```python
from build123d import *

# Parameters (mm, degrees)
SK_P01_P2020_R  = 2.1
P01_P2020_DEPTH = 120


with BuildPart() as part:
    # SK_P01_p2020 → P01_p2020 (new body)
    with BuildSketch(Plane(origin=(0, 0, 0), x_dir=(1, 0, 0), z_dir=(0, 1, 0))):
        Polygon((10, -10), (10, -3.1), (4, -3.1), (4, 3.1), (10, 3.1), (10, 10), (3.1, 10), (3.1, 4), (-3.1, 4), (-3.1, 10), (-10, 10), (-10, 3.1), (-4, 3.1), (-4, -3.1), (-10, -3.1), (-10, -10), (-3.1, -10), (-3.1, -4), (3.1, -4), (3.1, -10), align=None)
        with Locations(Location((0, 0, 0), (0, 0, 270))):
            Circle(SK_P01_P2020_R, mode=Mode.SUBTRACT)
    extrude(amount=P01_P2020_DEPTH)


solid = part.part
```
Here's how the part is built. I have some questions about the finished solid (model axes, mm). A direction names the side the tool comes from. Coordinates: 2 decimals unless noted, no trailing zeros. Order: outer loops, then holes, each group sorted by start corner. A loop starts at its lowest first (then second) coordinate and runs counter-clockwise, first axis right, second up. Notation, with made-up numbers: (55.5, 23) -> (90.5, 23) arc R30 cw to (90.5, 57) -> close; hole circle Ø1 at (-3, -37). An arc over 180 degrees is marked (long way). Return JSON: item names as keys, results as strings.
1) If we section it at B-B on z = -6.25: List the corners of the cut face in (x, y) for me.
Conclusion:
{"outline": "(-10, 0) -> (-3.1, 0) -> (-3.1, 120) -> (-10, 120) -> close; (3.1, 0) -> (10, 0) -> (10, 120) -> (3.1, 120) -> close"}
2) If I drill on probe 1 along Z at (x, y) = (-7.75, 58); probe 2 along X at (y, z) = (51.5, 0), over which ranges is the centre line in solid material (lowest first)?
Conclusion:
{"probe 1": "z = -10 to -3.1, 3.1 to 10", "probe 2": "x = -4 to -2.1, 2.1 to 4"}
3) If we section it at A-A on x = 0: List the corners of the cut face in (y, z) for me.
Conclusion:
{"outline": "(0, -4) -> (120, -4) -> (120, -2.1) -> (0, -2.1) -> close; (0, 2.1) -> (120, 2.1) -> (120, 4) -> (0, 4) -> close"}
4) If we section it at C-C on y = 79.5: List the corners of the cut face in (x, z) for me, plus the area to 3 significant figures.
Conclusion:
{"outline": "(-10, -10) -> (-3.1, -10) -> (-3.1, -4) -> (3.1, -4) -> (3.1, -10) -> (10, -10) -> (10, -3.1) -> (4, -3.1) -> (4, 3.1) -> (10, 3.1) -> (10, 10) -> (3.1, 10) -> (3.1, 4) -> (-3.1, 4) -> (-3.1, 10) -> (-10, 10) -> (-10, 3.1) -> (-4, 3.1) -> (-4, -3.1) -> (-10, -3.1) -> close; hole circle Ø4.2 at (0, 0)", "area": "237 mm²"}
5) Thinking about a two-plate mould opening in X: for faces 1 (the flat face through (-3.1, 59, -7)), 2 (the flat face through (-7, 59, -3.1)), 3 (the flat face through (-10, 59, 7)), which applies, +X half, -X half, draft (parallel to the pull), parting line (faces both ways), or undercut?
Conclusion:
{"face 1": "undercut", "face 2": "draft", "face 3": "-X half"}
6) I'm going to push flat-ended pins straight in: P1, Ø5, axis at y = 37, z = 0.5, coming from the +X side; P2, Ø1.5, axis at x = -1, y = 24, coming from the +Z side; P3, Ø3, axis at y = 58.5, z = 0, coming from the -X side. Where does each tip first touch, or does it pass through?
Conclusion:
{"P1": "stops at x = 4", "P2": "stops at z = 4", "P3": "stops at x = -4"}
7) On a 3-axis mill with a long thin cutter (end or side, diameter ignored), from which of +Z, -Z, +X, -X, +Y, -Y can I reach the whole of each face in a straight line? I mean faces 4 (the flat face through (0, 59, 4)), 5 (the flat face through (3.1, 59, -7)), 6 (the flat face through (-7, 59, 3.1)). Say none if no direction works.
Conclusion:
{"face 4": "+Z, +Y, -Y", "face 5": "-Z, +Y, -Y", "face 6": "-X, +Y, -Y"}
